from build123d import *

# Parameters (mm, degrees)
SKETCH1_W                = 40
SKETCH1_H                = 40
BOSS_EXTRUDE1_DEPTH      = 5
SKETCH2_R                = 20
BOSS_EXTRUDE2_DEPTH      = 20
BOSS_EXTRUDE3_DEPTH      = 5
SKETCH6_R                = 20
SKETCH6_R_2              = 16
EXTRUDE_THIN1_DEPTH      = 180
SKETCH7_W                = 32
SKETCH7_H                = 37
CUT_EXTRUDE1_DEPTH       = 16
BOSS_EXTRUDE4_DEPTH      = 0.5
BOSS_EXTRUDE4_DEPTH_BACK = 20
SKETCH8_W                = 8
SKETCH8_H                = 40
SKETCH12_W               = 40
SKETCH12_H               = 5
BOSS_EXTRUDE5_DEPTH      = 30
SKETCH10_W               = 13
SKETCH10_H               = 23
CUT_EXTRUDE2_DEPTH       = 20
SKETCH11_R               = 1.2
CUT_EXTRUDE3_DEPTH       = 10


with BuildPart() as part:
    # Sketch1 → Boss-Extrude1 (new body)
    with BuildSketch(Plane(origin=(0, 0, 0), x_dir=(1, 0, 0), z_dir=(0, 1, 0))):
        with Locations((20, -20)):
            Rectangle(SKETCH1_W, SKETCH1_H)
    extrude(amount=BOSS_EXTRUDE1_DEPTH)

    # Sketch2 → Boss-Extrude2 (add)
    with BuildSketch(Plane(origin=(0, 5, 0), x_dir=(1, 0, 0), z_dir=(0, 1, 0))):
        with Locations(Location((20, -20, 0), (0, 0, 270))):
            Circle(SKETCH2_R)
    extrude(amount=BOSS_EXTRUDE2_DEPTH)

    # Sketch4 → Boss-Extrude3 (add, symmetric)
    with BuildSketch(Plane.ZY.offset(-20)):
        Polygon((35, 25), (5, 25), (5, 32), align=None)
    extrude(amount=BOSS_EXTRUDE3_DEPTH, both=True)

    # Sketch6 → Extrude-Thin1 (add)
    with BuildSketch(Plane(origin=(0, 25, 0), x_dir=(1, 0, 0), z_dir=(0, 1, 0))):
        with Locations((20, -20)):
            Circle(SKETCH6_R)
        with Locations((20, -20)):
            Circle(SKETCH6_R_2, mode=Mode.SUBTRACT)
    extrude(amount=EXTRUDE_THIN1_DEPTH)

    # Sketch7 → Cut-Extrude1 (cut)
    with BuildSketch(Plane.XY.offset(40)):
        with Locations((20, 43.5)):
            Rectangle(SKETCH7_W, SKETCH7_H)
    extrude(amount=-CUT_EXTRUDE1_DEPTH, mode=Mode.SUBTRACT)

    # Sketch8 → Boss-Extrude4 (add, two sides: drawn at the far end of the back side and taken through both)
    with BuildSketch(Plane.ZY.offset(-36).offset(-BOSS_EXTRUDE4_DEPTH_BACK)):
        with Locations((28, 45)):
            Rectangle(SKETCH8_W, SKETCH8_H)
    extrude(amount=BOSS_EXTRUDE4_DEPTH + BOSS_EXTRUDE4_DEPTH_BACK)

    # Sketch12 → Boss-Extrude5 (add)
    with BuildSketch(Plane(origin=(0, 0, 0), x_dir=(-1, 0, 0), z_dir=(0, 0, -1))):
        with Locations((-20, 2.5)):
            Rectangle(SKETCH12_W, SKETCH12_H)
    extrude(amount=BOSS_EXTRUDE5_DEPTH)

    # Sketch10 → Cut-Extrude2 (cut)
    with BuildSketch(Plane.XY.offset(32)):
        with Locations((47, 44.5)):
            Rectangle(SKETCH10_W, SKETCH10_H)
    extrude(amount=-CUT_EXTRUDE2_DEPTH, mode=Mode.SUBTRACT)

    # Sketch11 → Cut-Extrude3 (cut)
    with BuildSketch(Plane.XY.offset(32)):
        with Locations((46.95, 30.4)):
            Circle(SKETCH11_R)
        with Locations((46.95, 58.1)):
            Circle(SKETCH11_R)
    extrude(amount=-CUT_EXTRUDE3_DEPTH, mode=Mode.SUBTRACT)


solid = part.part
Design review of the part built by this model. Coordinates are the model's own, in mm. A direction names the side the tool comes from. Coordinates: 2 decimals unless noted, no trailing zeros. Order: outer loops, then holes, each group sorted by start corner. A loop starts at its lowest first (then second) coordinate and runs counter-clockwise, first axis right, second up. Notation, with made-up numbers: (28, 29) - (35, 29) arc R27 ccw to (35, 66) - close; hole circle Ø11 at (8, -31.5). An arc over 180 degrees is marked (long way). Put each result on its own line as item: value.
1) Wall thickness on L1, parallel to Y at x = 4.5, z = 32.5; L2, parallel to X at y = 169, z = 20; L3, parallel to Y at x = 46.95, z = 30.25: over which ranges is each line inside the solid? List them lowest first. Write a range as from..to.
Response values:
L1: y = 0..25, 62..205
L2: x = 0..4, 36..40
L3: y = 25..29.2, 31.6..33, 56..56.9, 59.3..65
2) Take a section at B-B, the plane y = 185. Give the boundary of the cut face in (x, z), and give its area (3 significant figures).
Response values:
outline: circle Ø40 at (20, 20); hole circle Ø32 at (20, 20)
area: 452 mm²
3) Tool access review of faces 1 (the face through (17.917, 113.74, 4.136)), 2 (the face through (36, 5, 36)), 3 (the face through (40.5, 44, 28)): name each direction out of +Z, -Z, +X, -X, +Y, -Y from which nothing blocks a thin tool from reaching the whole face with its end or side.
Response values:
face 1: +Y
face 2: +Z, +X
face 3: +Z, -Z
4) Take a section at A-A, the plane x = 50. Give the boundary of the cut face in (y, z).
Response values:
outline: (25, 24) - (33, 24) - (33, 32) - (25, 32) - close; (56, 24) - (65, 24) - (65, 32) - (56, 32) - close
5) Insertion check: P1, Ø6.5, axis at x = 49, z = 28.5, coming from the -Y side; P2, Ø4, axis at x = 18.5, z = -21, coming from the +Y side; P3, Ø5, axis at x = 7, y = 56, coming from the -Z side. Each pin has a flat end and moves straight along its axis. Give the tip position at first contact, or say it passes through.
Response values:
P1: stops at y = 25
P2: stops at y = 5
P3: stops at z = 2.98
6) The part is to be moulded in two halves that separate along Y. For faces 4 (the face through (15, 28, 13)), 5 (the face through (35.5, 44, 28)), 6 (the face through (20, 5, -16)), say which applies: released by +Y, released by -Y, zero draft, split by the parting line, or undercut.
Response values:
face 4: zero draft
face 5: undercut
face 6: released by +Y
